Check sheet for the modelled part. Datum: model origin and axes. Units: mm. A direction names the side the tool comes from. Round coordinates to 2 decimals unless told otherwise and drop trailing zeros. Write each loop counter-clockwise with the first axis right and the second up, starting at its lowest first coordinate (ties: lowest second). Pieces come first, ordered by that corner, then holes. Notation, with made-up numbers: (41.5, 56.5) -> (75.5, 56.5) arc R14 cw to (75.5, 75.5) -> close; hole circle Ø11 at (21, 84). An arc over 180 degrees is marked (long way). Write item = value, one per line.
from build123d import *

# Parameters (mm, degrees)
SKETCH1_R           = 2.75
BOSS_EXTRUDE1_DEPTH = 2
SKETCH3_W           = 25
SKETCH3_H           = 12
BOSS_EXTRUDE2_DEPTH = 5
BOSS_EXTRUDE3_START = 2.5
SKETCH4_R           = 2.75
BOSS_EXTRUDE3_DEPTH = 2.5


with BuildPart() as part:
    # Sketch1 → Boss-Extrude1 (new body)
    with BuildSketch(Plane.YZ):
        with BuildLine():
            Line((0, 6), (45, 6))
            ThreePointArc((45, 6), (51, 0), (45, -6))
            Line((45, -6), (0, -6))
            ThreePointArc((0, -6), (-6, 0), (0, 6))
        make_face()
        with Locations(Location((0, 0, 0), (0, 0, 270))):
            Circle(SKETCH1_R, mode=Mode.SUBTRACT)
        with Locations(Location((45, 0, 0), (0, 0, 270))):
            Circle(SKETCH1_R, mode=Mode.SUBTRACT)
    extrude(amount=BOSS_EXTRUDE1_DEPTH)

    # Sketch3 → Boss-Extrude2 (add)
    with BuildSketch(Plane(origin=(0, 0, 0), x_dir=(0, -1, 0), z_dir=(-1, 0, 0))):
        with Locations((-22.5, 0)):
            Rectangle(SKETCH3_W, SKETCH3_H)
    extrude(amount=BOSS_EXTRUDE2_DEPTH)

    # Sketch4 → Boss-Extrude3 (add)
    with BuildSketch(Plane(origin=(-5, 0, 0), x_dir=(0, -1, 0), z_dir=(-1, 0, 0)).offset(BOSS_EXTRUDE3_START)):
        with BuildLine():
            Line((-45, 6), (0, 6))
            ThreePointArc((0, 6), (6, 0), (0, -6))
            Line((0, -6), (-45, -6))
            ThreePointArc((-45, -6), (-51, 0), (-45, 6))
        make_face()
        with Locations(Location((-45, 0, 0), (0, 0, 270))):
            Circle(SKETCH4_R, mode=Mode.SUBTRACT)
        with Locations(Location((0, 0, 0), (0, 0, 270))):
            Circle(SKETCH4_R, mode=Mode.SUBTRACT)
    extrude(amount=-BOSS_EXTRUDE3_DEPTH)


solid = part.part
(1) Sectioned sample at A-A on z = 0. Enter the section's corners in (x, y).
Worked answers:
outline = (-7.5, -6) -> (-5, -6) -> (-5, -2.75) -> (-7.5, -2.75) -> close; (-7.5, 2.75) -> (-5, 2.75) -> (-5, 10) -> (0, 10) -> (0, 2.75) -> (2, 2.75) -> (2, 42.25) -> (0, 42.25) -> (0, 35) -> (-5, 35) -> (-5, 42.25) -> (-7.5, 42.25) -> close; (-7.5, 47.75) -> (-5, 47.75) -> (-5, 51) -> (-7.5, 51) -> close; (0, -6) -> (2, -6) -> (2, -2.75) -> (0, -2.75) -> close; (0, 47.75) -> (2, 47.75) -> (2, 51) -> (0, 51) -> close
(2) Sectioned sample at C-C on x = -1.5. Enter the section's corners in (y, z).
Worked answers:
outline = (10, -6) -> (35, -6) -> (35, 6) -> (10, 6) -> close
(3) Material ranges on L1, parallel to Y at x = -6, z = 0; L2, parallel to Z at x = -6.3, y = 45; L3, parallel to X at y = 42.5, z = 4, recorded low to high. Write a range as [from, to].
Worked answers:
L1 = [-6, -2.75], [2.75, 42.25], [47.75, 51]
L2 = [-6, -2.75], [2.75, 6]
L3 = [-7.5, -5], [0, 2]
(4) Sectioned sample at B-B on x = 1.5. Enter the section's corners in (y, z), then the cut area to 3 significant figures.
Worked answers:
outline = (0, -6) -> (45, -6) arc R6 ccw to (45, 6) -> (0, 6) arc R6 ccw to start; hole circle Ø5.5 at (0, 0); hole circle Ø5.5 at (45, 0)
area = 606 mm²
(5) Release check for a two-part mould opening along Z. For faces 1 (the flat face through (-3, 22, -6)), 2 (the flat face through (-2, 10, 0)), 3 (the cylindrical face through (-6.268, 42.273, 0.358)) record: pulls with the +Z half, pulls with the -Z half, needs draft (parallel to the pull), parting line crosses it, or undercut.
Worked answers:
face_1 = pulls with the -Z half
face_2 = needs draft
face_3 = undercut
(6) Go/stop test with flat-tipped pins: P1, Ø3.5, axis at y = 0, z = 0, coming from the +X side; P2, Ø5.5, axis at x = -2, z = 2, coming from the +Y side; P3, Ø1.5, axis at x = -1.5, z = 1.5, coming from the +Y side. Record where each tip stops, or that it passes through.
Worked answers:
P1 = through
P2 = 51
P3 = 35
(7) Access from +Z, -Z, +X, -X, +Y, -Y to the whole of each face (thin tool, end or side, straight path). Record for faces 4 (the flat face through (-7.5, 22, 0)), 5 (the flat face through (0, 41, 0)), 6 (the flat face through (0, 4, 0)).
Worked answers:
face_4 = +Z, -Z, -X, +Y, -Y
face_5 = +Z, -Z, +Y
face_6 = +Z, -Z, -Y
